Here's how the part is built. I have some questions about the finished solid (model axes, mm). A direction names the side the tool comes from. Round coordinates to 2 decimals unless told otherwise and drop trailing zeros. Order: outer loops, then holes, each group sorted by start corner. A loop starts at its lowest first (then second) coordinate and runs counter-clockwise, first axis right, second up.
```python
from build123d import *

# Parameters (mm, degrees)
SKETCH1_W           = 63.5
SKETCH1_H           = 19.05
BOSS_EXTRUDE1_DEPTH = 6.35
SKETCH2_R           = 2.0955
SKETCH2_W           = 12.7
SKETCH2_H           = 6.35
CUT_EXTRUDE1_DEPTH  = 6.35
FILLET1_R           = 6.35


with BuildPart() as part:
    # Sketch1 → Boss-Extrude1 (new body)
    with BuildSketch(Plane.XY):
        Rectangle(SKETCH1_W, SKETCH1_H)
    extrude(amount=BOSS_EXTRUDE1_DEPTH)

    # Sketch2 → Cut-Extrude1 (cut)
    with BuildSketch(Plane.XY.offset(6.35)):
        Circle(SKETCH2_R)
        with Locations((-19.05, 0)):
            Rectangle(SKETCH2_W, SKETCH2_H)
        with Locations((19.05, 0)):
            Rectangle(SKETCH2_W, SKETCH2_H)
    extrude(amount=-CUT_EXTRUDE1_DEPTH, mode=Mode.SUBTRACT)

    # Fillet1
    fillet1_edges = [part.edges().sort_by_distance(p)[0] for p in [
        (31.75, -9.525, 3.175),
        (-31.75, -9.525, 3.175),
        (-31.75, 9.525, 3.175),
        (31.75, 9.525, 3.175),
    ]]
    fillet(fillet1_edges, radius=FILLET1_R)


solid = part.part
```
1) We'd pull the mould along X, two halves only. Please class faces 1 (the cylindrical face through (-29.939, -7.615, 3.219)), 2 (the flat face through (19, -3.175, 3)), 3 (the flat face through (31.75, 0, 3)): +X half, -X half, draft (parallel to the pull), parting line (faces both ways), or undercut.
2) If we section it at D-D (x = 19): Write out the boundary of the cut face in (y, z) (3 decimals), plus the area to 3 significant figures.
3) For faces 4 (the flat face through (-19, 3.175, 3)), 5 (the flat face through (-0.4, 2.3, 6.35)), which set-ups out of +Z, -Z, +X, -X, +Y, -Y let a thin tool reach every point of the face, with its end or its side?
4) If we section it at C-C (z = 2): Give the number of separate pieces and of enclosed holes in the cut face, plus the area to 4 significant figures.
5) I need wall thicknesses on line 1 (X direction, y = 3, z = 6); line 2 (Y direction, x = -19, z = 4.5) (3 decimals); line 3 (Y direction, x = 0, z = 4) (1 decimal). Which ranges of each line are inside material? Lowest first, please.
6) If we section it at B-B (y = 0): Write out the boundary of the cut face in (x, z).
7) I'm going to push flat-ended pins straight in: pin 1 (4 mm diameter, centred on x = 3.5, y = -2.5, fed in from -Z); pin 2 (2 mm diameter, centred on y = -5.5, z = 5.5, fed in from -X); pin 3 (3.5 mm diameter, centred on x = 0, y = 0, fed in from -Z). Where does each tip first touch, or does it pass through?
Solutions:
1. face 1: -X half
1. face 2: undercut
1. face 3: +X half
2. outline: (-9.525, 0) - (-3.175, 0) - (-3.175, 6.35) - (-9.525, 6.35) - close; (3.175, 0) - (9.525, 0) - (9.525, 6.35) - (3.175, 6.35) - close
2. area: 80.6 mm2
3. face 4: +Z, -Z
3. face 5: +Z, +X, -X, +Y, -Y
4. separate pieces: 1
4. enclosed holes: 3
4. area: 1,000 mm2
5. line 1: x = -31.75 to -25.4, -12.7 to 12.7, 25.4 to 31.75
5. line 2: y = -9.525 to -3.175, 3.175 to 9.525
5. line 3: y = -9.5 to -2.1, 2.1 to 9.5
6. outline: (-31.75, 0) - (-25.4, 0) - (-25.4, 6.35) - (-31.75, 6.35) - close; (-12.7, 0) - (-2.1, 0) - (-2.1, 6.35) - (-12.7, 6.35) - close; (2.1, 0) - (12.7, 0) - (12.7, 6.35) - (2.1, 6.35) - close; (25.4, 0) - (31.75, 0) - (31.75, 6.35) - (25.4, 6.35) - close
7. pin 1: stops at z = 0
7. pin 2: stops at x = -31.61
7. pin 3: passes through
